Could you check a few things on this drawing? It's one solid part, dimensions in mm from its lowest x, y, z. Give positions to 0.01 mm unless a question says otherwise; leave off trailing zeros. Write each loop counter-clockwise with the first axis right and the second up, starting at its lowest first coordinate (ties: lowest second). Pieces come first, ordered by that corner, then holes.
1. Suppose I cut it at B-B (y = 57.15). Please give me the cut outline in (x, z), and give its area (3 significant figures).
2. I'm going to push flat-ended pins straight in: pin 1 (3 mm diameter, centred on x = 148, y = 52, fed in from -Z); pin 2 (3.5 mm diameter, centred on x = 123.9, y = 57.15, fed in from -Z). Where does each tip first touch, or does it pass through?
3. Suppose I cut it at A-A (x = 123.9). Please give me the cut outline in (y, z), and give its area (3 significant figures).
4. If I drill on probe 1 along X at (y, z) = (57.15, 7.75); probe 2 along Y at (x, z) = (108.9, 8), over which ranges is the centre line in solid material (lowest first)?
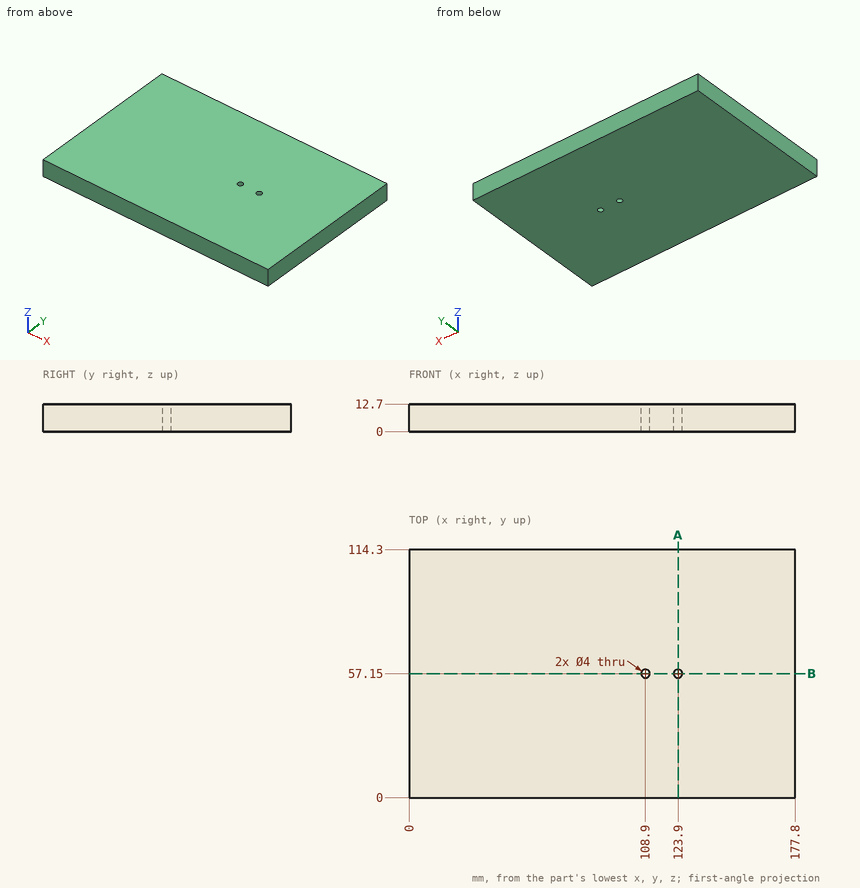
Checks:
1. outline: (0, 0) - (106.9, 0) - (106.9, 12.7) - (0, 12.7) - close; (110.9, 0) - (121.9, 0) - (121.9, 12.7) - (110.9, 12.7) - close; (125.9, 0) - (177.8, 0) - (177.8, 12.7) - (125.9, 12.7) - close
1. area: 2,160 mm2
2. pin 1: stops at z = 0
2. pin 2: passes through
3. outline: (0, 0) - (55.15, 0) - (55.15, 12.7) - (0, 12.7) - close; (59.15, 0) - (114.3, 0) - (114.3, 12.7) - (59.15, 12.7) - close
3. area: 1,400 mm2
4. probe 1: x = 0 to 106.9, 110.9 to 121.9, 125.9 to 177.8
4. probe 2: y = 0 to 55.15, 59.15 to 114.3
